The model under review builds one solid part; all positions refer to its coordinate system, in mm. Face numbers are marked on the shaded views. A direction names the side the tool comes from. Coordinates: 2 decimals unless noted, no trailing zeros. Write each loop counter-clockwise with the first axis right and the second up, starting at its lowest first coordinate (ties: lowest second). Pieces come first, ordered by that corner, then holes.
1) Add section A-A, the plane z = 9. State the section outline as (x, y) points.
2) Add section D-D, the plane z = 26.5. State the section outline as (x, y) points.
3) For line 1 (Y direction, x = 1.5, z = 15); line 2 (Z direction, x = -4.25, y = -6.25), list the stretches that pass through material, from the lowest coordinate up.
4) For P1, Ø5.5, axis at x = 2, z = 19, coming from the -Y side; P2, Ø6, axis at y = -3, z = 24, coming from the +X side; P3, Ø3, axis at x = -2, y = -6.5, coming from the +Z side, all flat-tipped, find the tip position at first contact; note any pin that passes through.
5) Add section B-B, the plane x = -8.5. State the section outline as (y, z) points, then the cut area to 3 significant figures.
6) Add section C-C, the plane y = -14. State the section outline as (x, z) points, then the cut area to 3 significant figures.
7) Machinability: for the marked faces 1, 2, 3 and 4, which of the approach directions +Z, -Z, +X, -X, +Y, -Y give a long, thin tool a straight path to every point of the face, cutting with its end or side? Answer none if there is none.
8) Mouldability with a two-part tool opening along Y and no side actions: class the marked faces 5, 6 and 7 as released by +Y, released by -Y, zero draft, split by the parting line, or undercut.
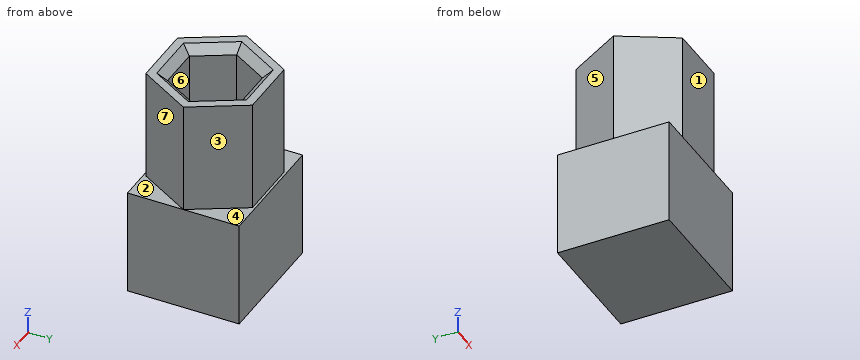
from build123d import *

# Parameters (mm, degrees)
SKETCH_W     = 22.05478
SKETCH_H     = 19.1
PAD_DEPTH    = 20
PAD001_DEPTH = 20
POCKET_DEPTH = 36.1
CHAMFER_SIZE = 1.5


with BuildPart() as part:
    # Sketch → Pad (new body)
    with BuildSketch(Plane.XZ):
        Rectangle(SKETCH_W, SKETCH_H)
    extrude(amount=PAD_DEPTH)

    # Sketch001 (on DatumPlane) → Pad001 (join)
    with BuildSketch(Plane(origin=(0, 0, 9.55), x_dir=(-1, 0, 0), z_dir=(0, 0, 1))):
        Polygon((-5.513695, 19.55), (-11.02739, 10), (-5.513695, 0.45), (5.513695, 0.45), (11.02739, 10), (5.513695, 19.55), align=None)
    extrude(amount=PAD001_DEPTH)

    # Sketch002 (on Face14 of Pad001) → Pocket (cut)
    with BuildSketch(Plane(origin=(0, 0, 29.55), x_dir=(-1, 0, 0), z_dir=(0, 0, 1))):
        Polygon((3.781644, 16.55), (-3.781644, 16.55), (-7.563289, 10), (-3.781644, 3.45), (3.781644, 3.45), (7.563289, 10), align=None)
    extrude(amount=-POCKET_DEPTH, mode=Mode.SUBTRACT)

    # Chamfer
    chamfer_edges = [part.edges().sort_by_distance(p)[0] for p in [
        (-5.672466, -6.725, 29.55),
        (-5.672466, -13.275, 29.55),
        (0, -3.45, 29.55),
        (5.672466, -6.725, 29.55),
        (5.672466, -13.275, 29.55),
        (0, -16.55, 29.55),
    ]]
    chamfer(chamfer_edges, length=CHAMFER_SIZE)


solid = part.part
Geometry results:
1. outline: (-11.03, -20) - (11.03, -20) - (11.03, 0) - (-11.03, 0) - close; hole (-7.56, -10) - (-3.78, -16.55) - (3.78, -16.55) - (7.56, -10) - (3.78, -3.45) - (-3.78, -3.45) - close
2. outline: (-11.03, -10) - (-5.51, -19.55) - (5.51, -19.55) - (11.03, -10) - (5.51, -0.45) - (-5.51, -0.45) - close; hole (-7.56, -10) - (-3.78, -16.55) - (3.78, -16.55) - (7.56, -10) - (3.78, -3.45) - (-3.78, -3.45) - close
3. line 1: y = -19.55 to -16.55, -3.45 to -0.45
3. line 2: z = -9.55 to -6.55
4. P1: stops at y = -19.55
4. P2: stops at x = 8.72
4. P3: stops at z = -6.55
5. outline: (-20, -9.55) - (0, -9.55) - (0, 9.55) - (-5.62, 9.55) - (-5.62, 29.55) - (-8.62, 29.55) - (-10, 28.86) - (-11.38, 29.55) - (-14.38, 29.55) - (-14.38, 9.55) - (-20, 9.55) - close
5. area: 556 mm2
6. outline: (-11.03, -9.55) - (11.03, -9.55) - (11.03, 9.55) - (8.72, 9.55) - (8.72, 29.55) - (6.99, 29.55) - (5.25, 28.05) - (5.25, -6.55) - (-5.25, -6.55) - (-5.25, 28.05) - (-6.99, 29.55) - (-8.72, 29.55) - (-8.72, 9.55) - (-11.03, 9.55) - close
6. area: 388 mm2
7. face 1: +Z, +X, -X, -Y
7. face 2: +Z, -Y
7. face 3: +Z, +X, +Y
7. face 4: +Z, +Y
8. face 5: released by +Y
8. face 6: undercut
8. face 7: released by -Y
